```python
from build123d import *

# Parameters (mm, degrees)
BOSS_EXTRUDE1_DEPTH = 10
SKETCH5_R           = 7.5
BOSS_EXTRUDE2_DEPTH = 15
SKETCH8_R           = 3.1
CUT_EXTRUDE1_DEPTH  = 9
CUT_EXTRUDE2_DEPTH  = 13


with BuildPart() as part:
    # Sketch4 → Boss-Extrude1 (new body)
    with BuildSketch(Plane.XY):
        with BuildLine():
            Line((-1.37, 5.27), (-1.37, 3.619392214))
            ThreePointArc((-1.37, 3.619392214), (0, -3.87), (1.37, 3.619392214))
            Line((1.37, 3.619392214), (1.37, 5.27))
            Line((1.37, 5.27), (-1.37, 5.27))
        make_face()
    extrude(amount=-BOSS_EXTRUDE1_DEPTH)

    # Sketch5 → Boss-Extrude2 (add)
    with BuildSketch(Plane.XY):
        Circle(SKETCH5_R)
    extrude(amount=BOSS_EXTRUDE2_DEPTH)

    # Sketch8 → Cut-Extrude1 (cut)
    with BuildSketch(Plane.XY.offset(15)):
        Circle(SKETCH8_R)
    extrude(amount=-CUT_EXTRUDE1_DEPTH, mode=Mode.SUBTRACT)

    # Sketch9 → Cut-Extrude2 (cut)
    with BuildSketch(Plane.XY.offset(15)):
        with BuildLine():
            Line((-3.1, 0), (0, 0))
            Line((0, 0), (3.1, 0))
            ThreePointArc((3.1, 0), (3.087680411, 0.276097227), (3.050819562, 0.55))
            Line((3.050819562, 0.55), (0, 0.55))
            Line((0, 0.55), (-3.050819562, 0.55))
            ThreePointArc((-3.050819562, 0.55), (-3.087680411, 0.276097227), (-3.1, 0))
        make_face()
        with BuildLine():
            Line((-6, 0), (-3.1, 0))
            ThreePointArc((-3.1, 0), (-3.087680411, 0.276097227), (-3.050819562, 0.55))
            Line((-3.050819562, 0.55), (-6, 0.55))
            Line((-6, 0.55), (-6, 0))
        make_face()
        with BuildLine():
            ThreePointArc((-3.050819562, -0.55), (-3.087680411, -0.276097227), (-3.1, 0))
            Line((-3.1, 0), (-6, 0))
            Line((-6, 0), (-6, -0.55))
            Line((-6, -0.55), (-3.050819562, -0.55))
        make_face()
        with BuildLine():
            Line((3.1, 0), (0, 0))
            Line((0, 0), (-3.1, 0))
            ThreePointArc((-3.1, 0), (-3.087680411, -0.276097227), (-3.050819562, -0.55))
            Line((-3.050819562, -0.55), (0, -0.55))
            Line((0, -0.55), (3.050819562, -0.55))
            ThreePointArc((3.050819562, -0.55), (3.087680411, -0.276097227), (3.1, 0))
        make_face()
        with BuildLine():
            Line((6, 0), (3.1, 0))
            ThreePointArc((3.1, 0), (3.087680411, -0.276097227), (3.050819562, -0.55))
            Line((3.050819562, -0.55), (6, -0.55))
            Line((6, -0.55), (6, 0))
        make_face()
        with BuildLine():
            ThreePointArc((3.050819562, 0.55), (3.087680411, 0.276097227), (3.1, 0))
            Line((3.1, 0), (6, 0))
            Line((6, 0), (6, 0.55))
            Line((6, 0.55), (3.050819562, 0.55))
        make_face()
    extrude(amount=-CUT_EXTRUDE2_DEPTH, mode=Mode.SUBTRACT)


solid = part.part
```
CAD build for the part. Positions are in the model's coordinates, mm. A direction names the side the tool comes from. Give positions to 0.01 mm unless a question says otherwise; leave off trailing zeros. Order: outer loops, then holes, each group sorted by start corner. A loop starts at its lowest first (then second) coordinate and runs counter-clockwise, first axis right, second up.
(1) Tool access for faces 4 (the flat face through (1.37, 4, -5)), 5 (the cylindrical face through (-0.151, -3.867, -4.93)), 6 (the flat face through (-1.37, 4, -5)), 7 (the flat face through (0.1, 0.55, 5.7)): list every direction of +Z, -Z, +X, -X, +Y, -Y with a clear straight run to the whole face (end or side of a thin tool).
(2) Saw through at D-D, the plane y = -1.75. Give the cut face in (x, z).
(3) Saw through at C-C, the plane z = -6.75. Give the cut face in (x, y), then the cut area to 3 significant figures.
(4) Saw through at A-A, the plane y = 0. Give the cut face in (x, z), then the cut area to 3 significant figures.
(5) Drill centre lines: L1, parallel to Y at x = -0.25, z = 5; L2, parallel to Z at x = -5, y = 0.5; L3, parallel to Z at x = -5.5, y = 1.5. Where is each one in solid material? Low to high.
(6) Mould opens along Y. For faces 1 (the flat face through (0, 5.27, -5)), 2 (the flat face through (2, -3, 15)), 3 (the flat face through (-6, 0, 9)) say: released by +Y, released by -Y, zero draft, split by the parting line, or undercut.
(7) Saw through at B-B, the plane x = 0. Give the cut face in (y, z), then the cut area to 3 significant figures.
(8) Flat gauge pins, fed straight in: pin 1 (2 mm diameter, centred on x = 0.5, z = -2.5, fed in from +Y); pin 2 (3 mm diameter, centred on x = 3, z = 8.5, fed in from +Y); pin 3 (1.5 mm diameter, centred on x = 4.5, z = 3.5, fed in from +Y). Where does each tip first touch, or does it go through?
Results found:
1. face 4: -Z, +X, +Y
1. face 5: -Z
1. face 6: -Z, -X, +Y
1. face 7: +Z
2. outline: (-7.29, 0) - (-3.45, 0) - (-3.45, -10) - (3.45, -10) - (3.45, 0) - (7.29, 0) - (7.29, 15) - (2.56, 15) - (2.56, 6) - (-2.56, 6) - (-2.56, 15) - (-7.29, 15) - close
3. outline: (-1.37, 3.62) arc R3.87 ccw (long way) to (1.37, 3.62) - (1.37, 5.27) - (-1.37, 5.27) - close
3. area: 51.1 mm2
4. outline: (-7.5, 0) - (-3.87, 0) - (-3.87, -10) - (3.87, -10) - (3.87, 0) - (7.5, 0) - (7.5, 15) - (6, 15) - (6, 2) - (-6, 2) - (-6, 15) - (-7.5, 15) - close
4. area: 146 mm2
5. L1: y = -7.5 to -0.55, 0.55 to 7.5
5. L2: z = 0 to 2
5. L3: z = 0 to 15
6. face 1: released by +Y
6. face 2: zero draft
6. face 3: undercut
7. outline: (-7.5, 0) - (-3.87, 0) - (-3.87, -10) - (5.27, -10) - (5.27, 0) - (7.5, 0) - (7.5, 15) - (3.1, 15) - (3.1, 6) - (0.55, 6) - (0.55, 2) - (-0.55, 2) - (-0.55, 6) - (-3.1, 6) - (-3.1, 15) - (-7.5, 15) - close
7. area: 256 mm2
8. pin 1: stops at y = 5.27
8. pin 2: stops at y = 7.35
8. pin 3: stops at y = 6.5
